Verification items for this drawing (mm, ordinates from the low corner). Round coordinates to 2 decimals unless told otherwise and drop trailing zeros. Order: outer loops, then holes, each group sorted by start corner. A loop starts at its lowest first (then second) coordinate and runs counter-clockwise, first axis right, second up.
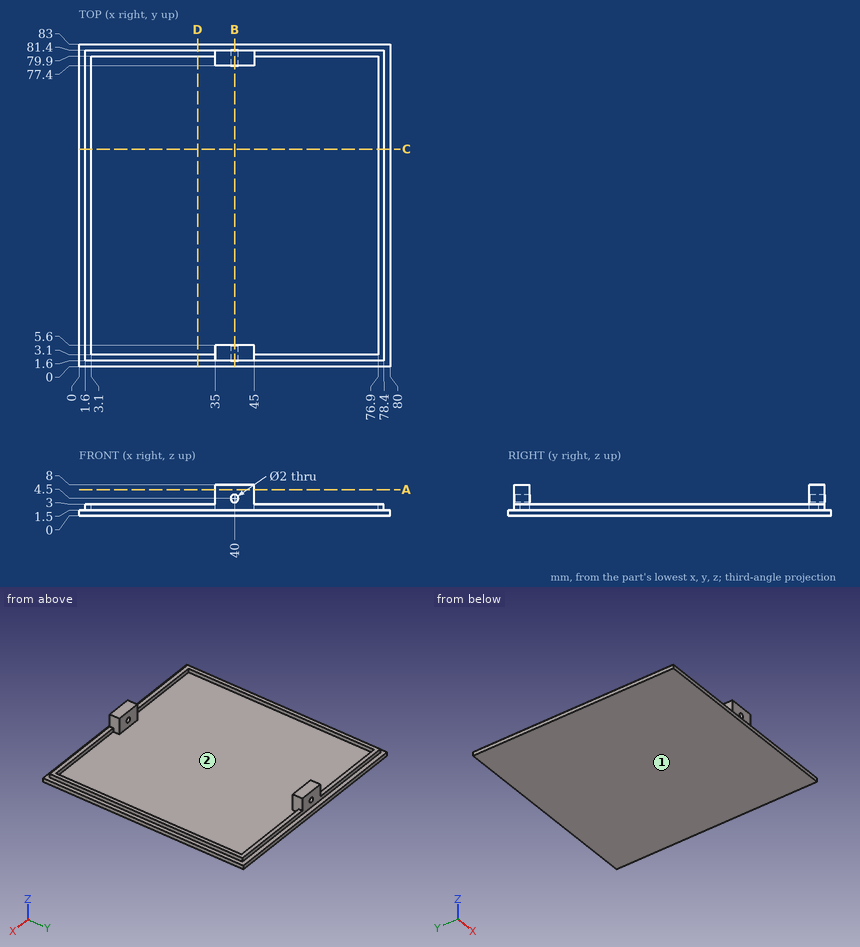
Item 1: Release check for a two-part mould opening along X. For the marked faces 1 and 2 record: released by +X, released by -X, zero draft, split by the parting line, or undercut.
Answer:
face 1: zero draft
face 2: undercut
Item 2: Sectioned sample at B-B (x = 40). Record the cut outline in (y, z).
Answer:
outline: (0, 0) - (83, 0) - (83, 1.5) - (81.4, 1.5) - (81.4, 3.5) - (77.4, 3.5) - (77.4, 1.5) - (5.6, 1.5) - (5.6, 3.5) - (1.6, 3.5) - (1.6, 1.5) - (0, 1.5) - close; (1.6, 5.5) - (5.6, 5.5) - (5.6, 8) - (1.6, 8) - close; (77.4, 5.5) - (81.4, 5.5) - (81.4, 8) - (77.4, 8) - close
Item 3: Sectioned sample at A-A (z = 6.75). Record the cut outline in (x, y), and give its area (3 significant figures).
Answer:
outline: (35, 1.6) - (45, 1.6) - (45, 5.6) - (35, 5.6) - close; (35, 77.4) - (45, 77.4) - (45, 81.4) - (35, 81.4) - close
area: 80.0 mm2
Item 4: Sectioned sample at D-D (x = 30.5). Record the cut outline in (y, z).
Answer:
outline: (0, 0) - (83, 0) - (83, 1.5) - (81.4, 1.5) - (81.4, 3) - (79.9, 3) - (79.9, 1.5) - (3.1, 1.5) - (3.1, 3) - (1.6, 3) - (1.6, 1.5) - (0, 1.5) - close
Item 5: Scan lines: line 1 along Y through (x, z) = (72, 2.75); line 2 along X through (y, z) = (21, 2.75); line 3 along Z through (x, y) = (40, 78.3). Record each from-to range of solid material in increasing order.
Answer:
line 1: y = 1.6 to 3.1, 79.9 to 81.4
line 2: x = 1.6 to 3.1, 76.9 to 78.4
line 3: z = 0 to 3.5, 5.5 to 8
Item 6: Sectioned sample at C-C (y = 56). Record the cut outline in (x, z).
Answer:
outline: (0, 0) - (80, 0) - (80, 1.5) - (78.4, 1.5) - (78.4, 3) - (76.9, 3) - (76.9, 1.5) - (3.1, 1.5) - (3.1, 3) - (1.6, 3) - (1.6, 1.5) - (0, 1.5) - close
Item 7: Go/stop test with flat-tipped pins: P1, Ø3, axis at x = 40.5, z = 3.5, coming from the +Y side; P2, Ø1.5, axis at x = 70, y = 52, coming from the +Z side; P3, Ø3, axis at x = 40, z = 4.5, coming from the -Y side. Record where each tip stops, or that it passes through.
Answer:
P1: stops at y = 81.4
P2: stops at z = 1.5
P3: stops at y = 1.6
